For this review, take the finished solid that the model builds, in its own axes (mm). A direction names the side the tool comes from. Coordinates: 2 decimals unless noted, no trailing zeros. Order: outer loops, then holes, each group sorted by start corner. A loop starts at its lowest first (then second) coordinate and runs counter-clockwise, first axis right, second up.
from build123d import *

# Parameters (mm, degrees)
F1_DEPTH = 63.5
F0_W     = 25.4
F0_H     = 19.05
F2_DEPTH = 63.5
F3_DEPTH = 7.9375
F5_R     = 5.08


with BuildPart() as f1:
    # F0 (on Front) → F1 (new body, symmetric)
    with BuildSketch(Plane.XZ):
        Polygon((-41.275, 9.525), (-41.275, -9.525), (41.275, -9.525), (41.275, 9.525), (22.225, 9.525), align=None)
    extrude(amount=F1_DEPTH, both=True)

    # F0 (on Front) → F2 (join, symmetric)
    with BuildSketch(Plane.XZ):
        with BuildLine():
            Line((22.225, 9.525), (41.275, 9.525))
            Line((41.275, 9.525), (41.275, 27.0002))
            ThreePointArc((41.275, 27.0002), (45.9246798487, 38.2255201513), (57.15, 42.8752))
            Line((57.15, 42.8752), (60.325, 42.8752))
            Line((60.325, 42.8752), (60.325, 61.9252))
            Line((60.325, 61.9252), (57.15, 61.9252))
            add(Edge.make_bspline(
                [(56.6897359672, 61.9221670411), (56.8432487019, 61.9234663989), (56.9966708454, 61.9244776876), (57.15, 61.9252)],
                knots=[111.1247319335, 111.1247319335, 111.1247319335, 111.1247319335, 111.5045361635, 111.5045361635, 111.5045361635, 111.5045361635], degree=3))
            ThreePointArc((56.6897359672, 61.9221670411), (32.2921003869, 51.5326367283), (22.225, 27.0002))
            Line((22.225, 27.0002), (22.225, 9.525))
        make_face()
        with Locations((73.025, 52.4002)):
            Rectangle(F0_W, F0_H)
    extrude(amount=F2_DEPTH, both=True)

    # F0 (on Front) → F3 (join, symmetric)
    with BuildSketch(Plane.XZ):
        with BuildLine():
            add(Edge.make_bspline(
                [(-41.275, 9.525), (-40.8962016322, 36.5015194538), (11.7743291488, 61.5419954401), (56.6897359672, 61.9221670411)],
                knots=[0, 0, 0, 0, 111.1247319335, 111.1247319335, 111.1247319335, 111.1247319335], degree=3))
            Line((-41.275, 9.525), (22.225, 9.525))
            Line((22.225, 9.525), (22.225, 27.0002))
            ThreePointArc((22.225, 27.0002), (32.2921003869, 51.5326367283), (56.6897359672, 61.9221670411))
        make_face()
    extrude(amount=F3_DEPTH, both=True)

    # F0 (on Front) → F4 (revolve)
    with BuildSketch(Plane.XZ):
        Polygon((85.725, 66.675), (85.725, 61.9252), (85.725, 42.8752), (85.725, 38.1), (111.125, 38.1), (111.125, 66.675), align=None)
    revolve(axis=Axis((85.725, 0, 52.3875), (0, 0, 1)))

    # F5
    f5_edges = [f1.edges().sort_by_distance(p)[0] for p in [
        (-41.275, -63.5, 0),
        (0, -63.5, -9.525),
        (41.275, -63.5, 8.7376),
        (45.92468, -63.5, 38.22552),
        (71.4375, -63.5, 42.8752),
        (85.725, -63.5, 52.4002),
        (71.4375, -63.5, 61.9252),
        (56.919867, -63.5, 61.923899),
        (32.2921, -63.5, 51.532637),
        (22.225, -63.5, 18.2626),
        (-9.525, -63.5, 9.525),
        (41.275, 63.5, 8.7376),
        (-41.275, 63.5, 0),
    ]]
    fillet(f5_edges, radius=F5_R)


solid = f1.part
1. Machinability: for faces 1 (the face through (71.24, 62.05, 44.4)), 2 (the face through (39.75, -62.05, 8.99)), 3 (the face through (-9, -34, 9.525)), 4 (the face through (41.275, -1, 8)), which of the approach directions +Z, -Z, +X, -X, +Y, -Y give a long, thin tool a straight path to every point of the face, cutting with its end or side? Answer none if there is none.
Answer below:
face 1: -Z, +X, +Y
face 2: -Z, +X, -Y
face 3: +Z, -X, -Y
face 4: -Z, +X, +Y, -Y
2. To check wall thickness, follow L1, parallel to Y at x = 0.5, z = 38.5; L2, parallel to X at y = -9, z = 13.5 (3 decimals); L3, parallel to Z at x = 10, y = -20.5 (3 decimals). State the ranges of each line that lie inside material, in increasing order.
Answer below:
L1: y = -7.94 to 7.94
L2: x = 22.225 to 41.275
L3: z = -9.525 to 9.525
3. Take a section at A-A, the plane x = 82.5. Give the boundary of the cut face in (y, z) (3 decimals), plus the area to 3 significant figures.
Answer below:
outline: (-63.149, 46.1) arc R5.08 ccw to (-58.42, 42.875) - (-25.194, 42.875) - (-25.194, 38.1) - (25.194, 38.1) - (25.194, 42.875) - (58.42, 42.875) arc R5.08 ccw to (63.5, 47.955) - (63.5, 61.925) - (25.194, 61.925) - (25.194, 66.675) - (-25.194, 66.675) - (-25.194, 61.925) - (-58.42, 61.925) arc R5.08 ccw to (-63.149, 58.7) - close
area: 2,880 mm2
4. Take a section at B-B, the plane z = 6.5. Give the boundary of the cut face in (x, y) (3 decimals).
Answer below:
outline: (-41.275, -58.42) arc R5.08 ccw to (-38.25, -63.066) - (25.25, -63.066) arc R5.08 ccw to (27.305, -63.5) - (36.195, -63.5) arc R5.08 ccw to (41.275, -58.42) - (41.275, 58.42) arc R5.08 ccw to (36.195, 63.5) - (-36.195, 63.5) arc R5.08 ccw to (-41.275, 58.42) - close
5. Clearance check with flat-ended pins moving along their axes: pin 1 Ø5 at (y, z) = (-6, 19.5) entering from +X (3 decimals); pin 2 Ø8.5 at (y, z) = (-27.5, 17.5) entering from -X (3 decimals); pin 3 Ø23 at (x, y) = (65, -26.5) entering from -Z. State where each tip first meets the part, or that it passes through.
Answer below:
pin 1: stops at x = 41.275
pin 2: stops at x = 22.225
pin 3: stops at z = 38.1
